Input: part model. Units: mm. Frame: model coordinates. Face numbers are marked on the shaded views. A direction names the side the tool comes from. Round coordinates to 2 decimals unless told otherwise and drop trailing zeros. Write each loop counter-clockwise with the first axis right and the second up, starting at its lowest first coordinate (ties: lowest second). Pieces come first, ordered by that corner, then holes. Notation, with made-up numbers: (7.25, 43) -> (65.25, 43) arc R22 cw to (65.25, 70) -> close; hole circle Ø9 at (42.5, -34.5). An arc over 180 degrees is marked (long way). Write item = value, one per line.
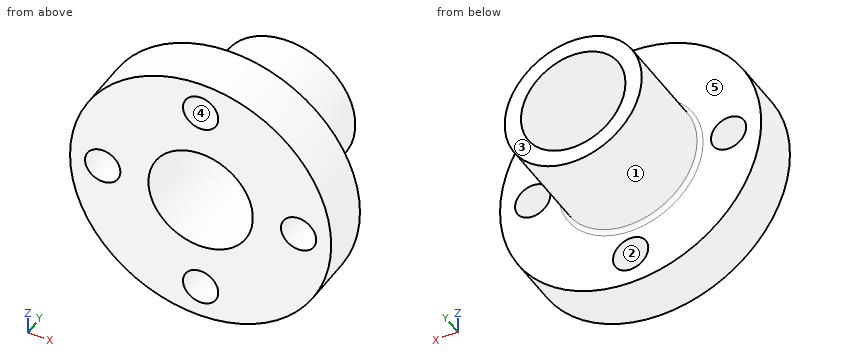
```python
from build123d import *

# Parameters (mm, degrees)
SKETCH3_R          = 1.35
CUT_EXTRUDE1_DEPTH = 10
FILLET1_R          = 0.3


with BuildPart() as part:
    # Sketch2 → Revolve1 (revolve)
    with BuildSketch(Plane.XY, mode=Mode.PRIVATE) as revolve1_sk:
        Polygon((4, 12), (4, 0), (10, 0), (10, 4), (5.25, 4), (5.25, 12), align=None)
    revolve(revolve1_sk.sketch.rotate(Axis((0, 12, 0), (0, -1, 0)), 180), axis=Axis((0, 12, 0), (0, -1, 0)))

    # Sketch3 → Cut-Extrude1 (cut)
    with BuildSketch(Plane(origin=(0, 4, 0), x_dir=(1, 0, 0), z_dir=(0, 1, 0))):
        with Locations(Location((7.5, 0, 0), (0, 0, 180))):
            Circle(SKETCH3_R)
        with Locations(Location((0, -7.5, 0), (0, 0, 180))):
            Circle(SKETCH3_R)
        with Locations(Location((-7.5, 0, 0), (0, 0, 180))):
            Circle(SKETCH3_R)
        with Locations(Location((0, 7.5, 0), (0, 0, 180))):
            Circle(SKETCH3_R)
    extrude(amount=-CUT_EXTRUDE1_DEPTH, mode=Mode.SUBTRACT)

    # Fillet1
    fillet1_edges = [part.edges().sort_by_distance(p)[0] for p in [
        (5.25, 4, 0),
    ]]
    fillet(fillet1_edges, radius=FILLET1_R)


solid = part.part
```
1) Cut plane A-A (z = 7.5). Return the cut outline in (x, y), and give its area (3 significant figures).
Solutions:
outline = (-6.61, 0) -> (-1.35, 0) -> (-1.35, 4) -> (-6.61, 4) -> close; (1.35, 0) -> (6.61, 0) -> (6.61, 4) -> (1.35, 4) -> close
area = 42.1 mm^2
2) Cut plane B-B (x = 7.5). Return the cut outline in (y, z).
Solutions:
outline = (0, -6.61) -> (4, -6.61) -> (4, -1.35) -> (0, -1.35) -> close; (0, 1.35) -> (4, 1.35) -> (4, 6.61) -> (0, 6.61) -> close
3) Draft query along X for the marked faces 1, 2 and 3. Return one class per face: +X half, -X half, draft (parallel to the pull), parting line (faces both ways), or undercut.
Solutions:
face_1 = parting line
face_2 = undercut
face_3 = draft
4) Line query: L1, parallel to Z at x = 0, y = 2.45; L2, parallel to Z at x = 0, y = 10.75; L3, parallel to Y at x = 5.75, z = -6.25. Output: solid intervals per line, ascending. Write a range as from..to.
Solutions:
L1 = -10..-8.85, -6.15..-4, 4..6.15, 8.85..10
L2 = -5.25..-4, 4..5.25
L3 = 0..4
5) Cut plane C-C (y = 2.5). Return the cut outline in (x, z).
Solutions:
outline = circle Ø20 at (0, 0); hole circle Ø2.7 at (-7.5, 0); hole circle Ø8 at (0, 0); hole circle Ø2.7 at (0, -7.5); hole circle Ø2.7 at (0, 7.5); hole circle Ø2.7 at (7.5, 0)
6) First-contact query: P1, Ø2, axis at y = 7, z = -1.5, coming from the +X side; P2, Ø4, axis at y = 5.5, z = -4, coming from the -X side (3 decimals). Flat tips, straight axial feed; report the tip coordinate or a pass-through.
Solutions:
P1 = 5.23
P2 = -9.635
7) Access query for the marked faces 4 and 5. Directions: +Z, -Z, +X, -X, +Y, -Y. A direction counts if a zero-diameter tool reaches every point of the face in a straight line with its end or side. Return the directions, or none.
Solutions:
face_4 = +Y, -Y
face_5 = +Y
8) Cut plane D-D (y = 8). Return the cut outline in (x, z).
Solutions:
outline = circle Ø10.5 at (0, 0); hole circle Ø8 at (0, 0)
